from build123d import *

# Parameters (mm, degrees)
EXTRUDE_1_DEPTH = 10
M2X0_4_1_D      = 1.6
M2X0_4_2_D      = 1.6


with BuildPart() as part:
    # ｽｹｯﾁ2 → ﾎﾞｽ - 押し出し1 (new body)
    with BuildSketch(Plane.XY):
        with BuildLine():
            ThreePointArc((-20, 0), (-22.928932188, 7.071067812), (-30, 10))
            Line((-30, 10), (-30, 1.05))
            ThreePointArc((-30, 1.05), (-29.25753788, 0.74246212), (-28.95, 0))
            ThreePointArc((-28.95, 0), (-29.25753788, -0.74246212), (-30, -1.05))
            Line((-30, -1.05), (-30, -10))
            ThreePointArc((-30, -10), (-22.928932188, -7.071067812), (-20, 0))
        make_face()
        with BuildLine():
            Line((-30, 1.05), (-30, 10))
            ThreePointArc((-30, 10), (-40, 0), (-30, -10))
            Line((-30, -10), (-30, -1.05))
            ThreePointArc((-30, -1.05), (-31.05, 0), (-30, 1.05))
        make_face()
        with BuildLine():
            Line((30, 10), (-30, 10))
            ThreePointArc((-30, 10), (-22.928932188, 7.071067812), (-20, 0))
            ThreePointArc((-20, 0), (-22.928932188, -7.071067812), (-30, -10))
            Line((-30, -10), (30, -10))
            ThreePointArc((30, -10), (20, 0), (30, 10))
        make_face()
        with BuildLine():
            ThreePointArc((40, 0), (37.071067812, 7.071067812), (30, 10))
            Line((30, 10), (30, 1.05))
            ThreePointArc((30, 1.05), (30.74246212, 0.74246212), (31.05, 0))
            ThreePointArc((31.05, 0), (30.74246212, -0.74246212), (30, -1.05))
            Line((30, -1.05), (30, -10))
            ThreePointArc((30, -10), (37.071067812, -7.071067812), (40, 0))
        make_face()
        with BuildLine():
            Line((30, 1.05), (30, 10))
            ThreePointArc((30, 10), (20, 0), (30, -10))
            Line((30, -10), (30, -1.05))
            ThreePointArc((30, -1.05), (28.95, 0), (30, 1.05))
        make_face()
    extrude(amount=EXTRUDE_1_DEPTH)

    # M2x0.4 ねじ穴1 (through all)
    with Locations(Plane.XY.offset(10)):
        with Locations((-30, 7.2), (-37.2, 0), (-30, -7.2)):
            Hole(M2X0_4_1_D / 2)

    # M2x0.4 ねじ穴2 (through all)
    with Locations(Plane.XY.offset(10)):
        with Locations((-22.8, 0)):
            Hole(M2X0_4_2_D / 2)


solid = part.part
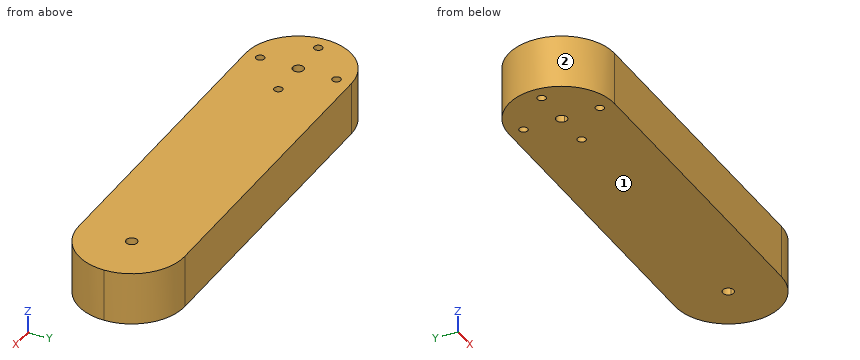
Read the model definition and answer for the solid it produces. Units are mm, in the model's axes. Face numbers are marked on the shaded views. Give positions to 0.01 mm unless a question says otherwise; leave off trailing zeros. Write each loop counter-clockwise with the first axis right and the second up, starting at its lowest first coordinate (ties: lowest second). Pieces come first, ordered by that corner, then holes. Notation, with made-up numbers: (44, 20.25) - (77, 20.25) arc R24 ccw to (77, 49.25) - close; hole circle Ø1 at (-15.5, 52.5). An arc over 180 degrees is marked (long way). Answer in a Markdown table with one row per item. Add a question column.
Item 1: Section D-D, the plane x = -32 is taken. Write down the section's boundary in (y, z), and give its area (3 significant figures).
Item 2: Section B-B, the plane z = 8 is taken. Write down the section's boundary in (x, y), and give its area (3 significant figures).
Item 3: Flat-ended cylindrical pins translate along their axes: P1, Ø6, axis at y = 8, z = 7.5, coming from the +X side; P2, Ø1, axis at y = 6.5, z = 4, coming from the +X side; P3, Ø2, axis at y = 5, z = 2.5, coming from the +X side; P4, Ø2, axis at x = 11, y = 5.5, coming from the -Z side. Find the tip coordinate at first contact, or state that the pin passes through.
Item 4: Determine the mould class of the marked faces 1 and 2 for opening direction X: pulls with the +X half, pulls with the -X half, needs draft (parallel to the pull), parting line crosses it, or undercut.
Item 5: Section A-A, the plane x = -22.8 is taken. Write down the section's boundary in (y, z), and give its area (3 significant figures).
Item 6: Section C-C, the plane y = -7.2 is taken. Write down the section's boundary in (x, z), and give its area (3 significant figures).
Item 7: Find the intervals of material crossed by L1, parallel to Y at x = -30, z = 4.5; L2, parallel to Y at x = -22.8, z = 4.75; L3, parallel to X at y = 6.75, z = 5.25, in increasing order.
Recorded:
| question | item | result |
|---|---|---|
| 1 | outline | (-9.8, 0) - (9.8, 0) - (9.8, 10) - (-9.8, 10) - close |
| 1 | area | 196 mm2 |
| 2 | outline | (-30, -10) - (30, -10) arc R10 ccw to (30, 10) - (-30, 10) arc R10 ccw to start; hole circle Ø1.6 at (-37.2, 0); hole circle Ø2.1 at (-30, 0); hole circle Ø1.6 at (-30, -7.2); hole circle Ø1.6 at (-30, 7.2); hole circle Ø1.6 at (-22.8, 0); hole circle Ø2.1 at (30, 0) |
| 2 | area | 1,500 mm2 |
| 3 | P1 | stops at x = 38.66 |
| 3 | P2 | stops at x = 38 |
| 3 | P3 | stops at x = 39.17 |
| 3 | P4 | stops at z = 0 |
| 4 | face 1 | needs draft |
| 4 | face 2 | pulls with the -X half |
| 5 | outline | (-10, 0) - (-0.8, 0) - (-0.8, 10) - (-10, 10) - close; (0.8, 0) - (10, 0) - (10, 10) - (0.8, 10) - close |
| 5 | area | 184 mm2 |
| 6 | outline | (-36.94, 0) - (-30.8, 0) - (-30.8, 10) - (-36.94, 10) - close; (-29.2, 0) - (36.94, 0) - (36.94, 10) - (-29.2, 10) - close |
| 6 | area | 723 mm2 |
| 7 | L1 | y = -10 to -8, -6.4 to -1.05, 1.05 to 6.4, 8 to 10 |
| 7 | L2 | y = -10 to -0.8, 0.8 to 10 |
| 7 | L3 | x = -37.38 to -30.66, -29.34 to 37.38 |
